Verification items for the finished model (mm, model axes). A direction names the side the tool comes from. Coordinates: 2 decimals unless noted, no trailing zeros. Loops run counter-clockwise (first coordinate to the right, second up) from the corner with the lowest first, then second, coordinate; pieces in that order, holes last. Notation, with made-up numbers: (43, 20.5) - (49, 20.5) arc R26 ccw to (49, 44.5) - close; hole circle Ø10 at (-37.5, 30). An arc over 180 degrees is marked (long way). Answer as CSV lines item,"result". Start each with the question number.
1. Cross-section at A-A (z = 0). Enter the section's corners in (x, y).
2. Cross-section at B-B (y = 24). Enter the section's corners in (x, z).
3. Material ranges on line 1 (Y direction, x = -16, z = 15); line 2 (Y direction, x = -15, z = 11); line 3 (X direction, y = 17.5, z = 0), recorded low to high. Write a range as [from, to].
4. Release check for a two-part mould opening along Z. For faces 4 (the flat face through (22.5, 22, 2)), 5 (the cylindrical face through (0, 22, 8)), 6 (the flat face through (-21.5, 22.2, 19)) record: pulls with the +Z half, pulls with the -Z half, needs draft (parallel to the pull), parting line crosses it, or undercut.
5. Gauge pin test, flat ends, axial feed: P1, Ø5, axis at x = -7.5, y = 14, coming from the +Z side; P2, Ø4.5, axis at x = 16, y = 37.5, coming from the +Z side. Record the tip position at first contact, or that the pin passes through.
6. Set-up check for faces 1 (the flat face through (3.5, 22.2, 19)), 2 (the flat face through (7.176, 22.185, -9.753)), 3 (the cylindrical face through (15.46, 35.06, 14.08)): record each of +Z, -Z, +X, -X, +Y, -Y from which the full face is reachable in a straight line by a thin tool's end or side.
7. Cross-section at D-D (z = -5.5). Enter the section's corners in (x, y).
8. Cross-section at C-C (x = 16). Enter the section's corners in (y, z), plus the area to 4 significant figures.
```python
from build123d import *

# Parameters (mm, degrees)
F1_DEPTH = 45
F3_SIZE  = 2
F2_R     = 2.5
F4_DEPTH = 12


with BuildPart() as f1:
    # F0 (on Front) → F1 (new body)
    with BuildSketch(Plane.XZ):
        with BuildLine():
            ThreePointArc((-4.526972, -6.595947), (0, 8), (4.526972, -6.595947))
            Line((4.526972, -6.595947), (9.900611, -13))
            Line((9.900611, -13), (22.5, -13))
            Line((22.5, -13), (22.5, 20))
            Line((22.5, 20), (12.5, 20))
            Line((12.5, 20), (10.5, 18))
            Line((10.5, 18), (4.5, 18))
            Line((4.5, 18), (2.5, 20))
            Line((2.5, 20), (0, 20))
            Line((0, 20), (-2.5, 20))
            Line((-2.5, 20), (-4.5, 18))
            Line((-4.5, 18), (-10.5, 18))
            Line((-10.5, 18), (-12.5, 20))
            Line((-12.5, 20), (-22.5, 20))
            Line((-22.5, 20), (-22.5, -13))
            Line((-22.5, -13), (-9.900611, -13))
            Line((-9.900611, -13), (-4.526972, -6.595947))
        make_face()
    extrude(amount=-F1_DEPTH)

    # F3
    f3_edges = [f1.edges().sort_by_distance(p)[0] for p in [
        (22.5, 22.5, 20),
        (-22.5, 22.5, 20),
    ]]
    chamfer(f3_edges, length=F3_SIZE)

    # F2 (on face) → F4 (cut)
    with BuildSketch(Plane.XY.offset(20)):
        with Locations((-16, 37.5)):
            Circle(F2_R)
        with Locations((-16, 7.5)):
            Circle(F2_R)
        with Locations((16, 37.5)):
            Circle(F2_R)
        with Locations((16, 7.5)):
            Circle(F2_R)
    extrude(amount=-F4_DEPTH, mode=Mode.SUBTRACT)


solid = f1.part
```
Values follow:
1,outline,"(-22.5, 0) - (-8, 0) - (-8, 45) - (-22.5, 45) - close; (8, 0) - (22.5, 0) - (22.5, 45) - (8, 45) - close"
2,outline,"(-22.5, -13) - (-9.9, -13) - (-4.53, -6.6) arc R8 cw (long way) to (4.53, -6.6) - (9.9, -13) - (22.5, -13) - (22.5, 18) - (20.5, 20) - (12.5, 20) - (10.5, 18) - (4.5, 18) - (2.5, 20) - (-2.5, 20) - (-4.5, 18) - (-10.5, 18) - (-12.5, 20) - (-20.5, 20) - (-22.5, 18) - close"
3,line 1,"y = [0, 5], [10, 35], [40, 45]"
3,line 2,"y = [0, 5.21], [9.79, 35.21], [39.79, 45]"
3,line 3,"x = [-22.5, -8], [8, 22.5]"
4,face 4,"needs draft"
4,face 5,"undercut"
4,face 6,"pulls with the +Z half"
5,P1,"stops at z = 18"
5,P2,"stops at z = 8"
6,face 1,"+Z, +Y, -Y"
6,face 2,"-Z, +Y, -Y"
6,face 3,"+Z"
7,outline,"(-22.5, 0) - (-5.81, 0) - (-5.81, 45) - (-22.5, 45) - close; (5.81, 0) - (22.5, 0) - (22.5, 45) - (5.81, 45) - close"
8,outline,"(0, -13) - (45, -13) - (45, 20) - (40, 20) - (40, 8) - (35, 8) - (35, 20) - (10, 20) - (10, 8) - (5, 8) - (5, 20) - (0, 20) - close"
8,area,"1,365 mm²"
